Answer from the drawing. Dimensions are ordinates in mm from the lowest x, y and z of the part. A direction names the side the tool comes from. Give positions to 0.01 mm unless a question says otherwise; leave off trailing zeros. Order: outer loops, then holes, each group sorted by start corner. A loop starts at its lowest first (then second) coordinate and runs counter-clockwise, first axis right, second up. Notation, with made-up numbers: (-7.75, -17) - (6.25, -17) arc R17 cw to (6.25, -12) - close; hole circle Ø10 at (76.5, 66). An arc over 180 degrees is marked (long way). One line per item, written item: value. Start each with the question number.
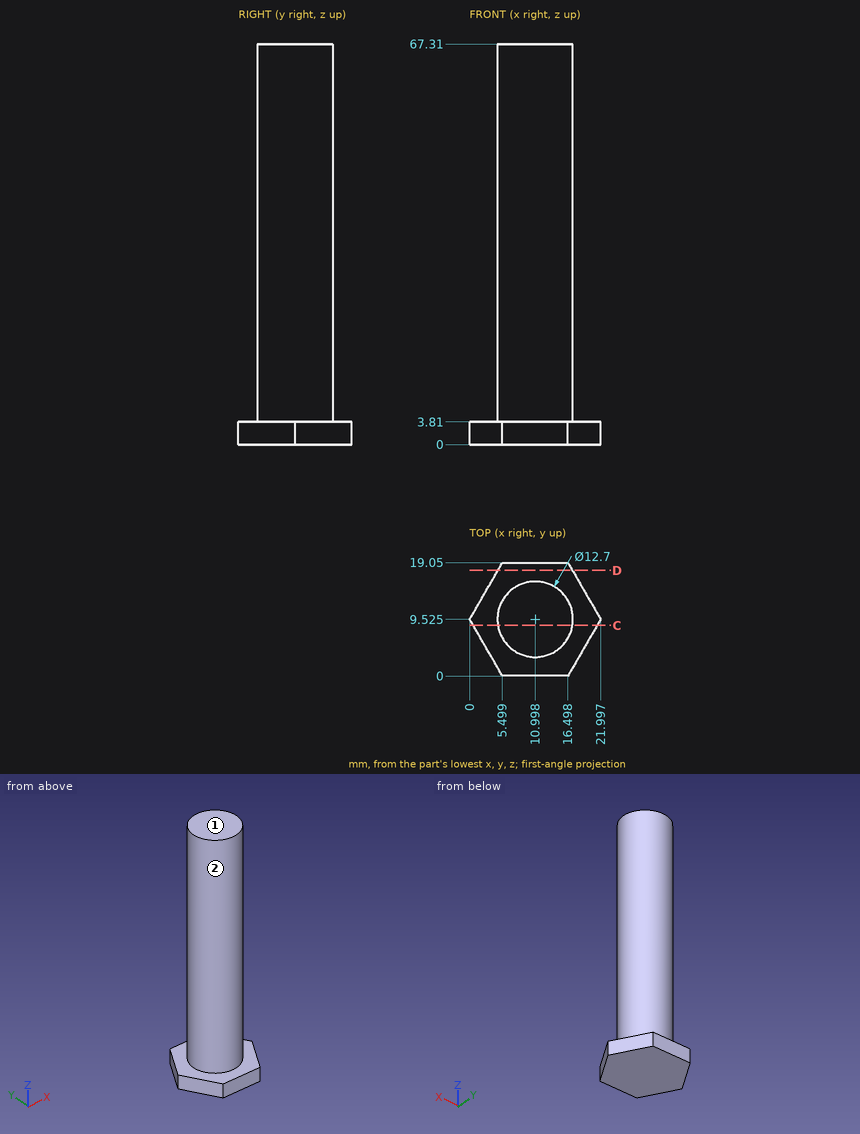
1) Section C-C on y = 8.5 is taken. Write down the section's boundary in (x, z) (1 decimal), plus the area to 3 significant figures.
2) Section D-D on y = 17.75 is taken. Write down the section's boundary in (x, z).
3) Each of these flat-tipped pins is pushed along its axis until it touches: pin 1 (1 mm diameter, centred on y = 5, z = 13.5, fed in from +X); pin 2 (6 mm diameter, centred on x = 19.5, z = 31.5, fed in from -Y) (1 decimal); pin 3 (4 mm diameter, centred on y = 11.5, z = 49.5, fed in from -X). Where does it stop, or does it pass through?
4) Find the intervals of material crossed by probe 1 along Z at (x, y) = (5.5, 15); probe 2 along Y at (x, z) = (13, 30.5); probe 3 along Y at (x, z) = (10.25, 13), in increasing order. Write a range as from..to.
5) For the marked faces 1 and 2, determine the directions among +Z, -Z, +X, -X, +Y, -Y from which every point of the face is accessible in a straight line to the end or side of a thin tool.
Solved:
1. outline: (0.6, 0) - (21.4, 0) - (21.4, 3.8) - (17.3, 3.8) - (17.3, 67.3) - (4.7, 67.3) - (4.7, 3.8) - (0.6, 3.8) - close
1. area: 875 mm2
2. outline: (4.75, 0) - (17.25, 0) - (17.25, 3.81) - (4.75, 3.81) - close
3. pin 1: stops at x = 15.91
3. pin 2: stops at y = 6.4
3. pin 3: stops at x = 4.65
4. probe 1: z = 0..3.81
4. probe 2: y = 3.5..15.55
4. probe 3: y = 3.22..15.83
5. face 1: +Z, +X, -X, +Y, -Y
5. face 2: +Z
